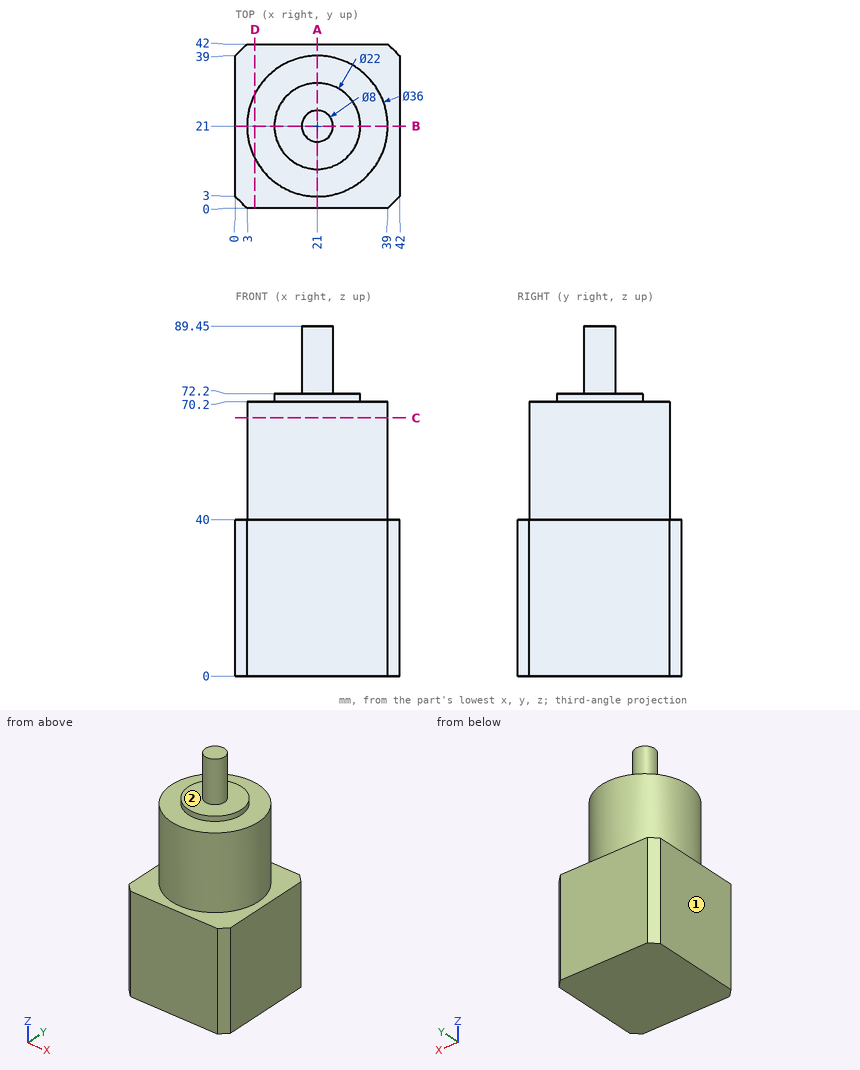
Can you work these out from the drawing? Everything is in mm from the part's minimum corner. A direction names the side the tool comes from. Round coordinates to 2 decimals unless told otherwise and drop trailing zeros. Loops run counter-clockwise (first coordinate to the right, second up) from the corner with the lowest first, then second, coordinate; pieces in that order, holes last. Notation, with made-up numbers: M 79,50 L 115,50 A20 cw 115,62 Z; hole C 40.5,-7 d9. An arc over 180 degrees is marked long. Answer in a Markdown table with one row per item.
1. I'm going to push flat-ended pins straight in: pin 1 Ø2 at (x, y) = (21, 15) entering from +Z; pin 2 Ø8 at (x, z) = (26.5, 15.5) entering from -Y; pin 3 Ø12 at (x, z) = (22.5, 76.5) entering from -Y; pin 4 Ø1 at (x, z) = (15.5, 74) entering from +Y. Where does each tip first touch, or does it pass through?
Established:
| item | result |
|---|---|
| pin 1 | z = 72.2 |
| pin 2 | y = 0 |
| pin 3 | y = 10 |
| pin 4 | through |
2. If we section it at A-A, the plane x = 21: Please give me the cut outline in (y, z).
Established:
| item | result |
|---|---|
| outline | M 0,0 L 42,0 L 42,40 L 39,40 L 39,70.2 L 32,70.2 L 32,72.2 L 25,72.2 L 25,89.45 L 17,89.45 L 17,72.2 L 10,72.2 L 10,70.2 L 3,70.2 L 3,40 L 0,40 Z |
3. If we section it at C-C, the plane z = 66: Please give me the cut outline in (x, y), plus the area to 3 significant figures.
Established:
| item | result |
|---|---|
| outline | C 21,21 d36 |
| area | 1,020 mm² |
4. Please list where these lines run through material, in increasing order: line 1 (Z direction, x = 23.5, y = 31); line 2 (Z direction, x = 18, y = 9.5); line 3 (Y direction, x = 7.5, z = 46). Write a range as from..to.
Established:
| item | result |
|---|---|
| line 1 | 0..72.2 |
| line 2 | 0..70.2 |
| line 3 | 9.09..32.91 |
5. If we section it at D-D, the plane x = 5: Please give me the cut outline in (y, z), plus the area to 3 significant figures.
Established:
| item | result |
|---|---|
| outline | M 0,0 L 42,0 L 42,40 L 29.25,40 L 29.25,70.2 L 12.75,70.2 L 12.75,40 L 0,40 Z |
| area | 2,180 mm² |
6. On a 3-axis mill with a long thin cutter (end or side, diameter ignored), from which of +Z, -Z, +X, -X, +Y, -Y can I reach the whole of each face in a straight line? I mean the marked faces 1 and 2. Say none if no direction works.
Established:
| item | result |
|---|---|
| face 1 | +Z, -Z, -X, +Y, -Y |
| face 2 | +Z |
